Can you work these out from the drawing? Everything is in mm from the part's minimum corner. Round coordinates to 2 decimals unless told otherwise and drop trailing zeros. Write each loop counter-clockwise with the first axis right and the second up, starting at its lowest first coordinate (ties: lowest second). Pieces come first, ordered by that corner, then holes. Notation, with made-up numbers: (28.5, -6) -> (80.5, -6) arc R28 ccw to (80.5, 32) -> close; hole circle Ø11 at (82, 16.25). An arc over 180 degrees is marked (long way). One line per question, with ' | ' between items. Start each with the question number.
1. Imagine slicing it at B-B, the plane y = 5.75. List the corners of the cut face in (x, z) for me.
2. For pin 1 Ø4 at (x, y) = (10.5, 6.5) entering from +Z, with a flat end and sliding along its axis, tell me the tip position at first contact or that it passes through.
3. If I drill on line 1 along X through (y, z) = (6.25, 0.65) (1 decimal); line 2 along Y through (x, z) = (6.25, 0.7) (1 decimal); line 3 along X through (y, z) = (5, 0.6), over which ranges is the centre line in solid material (lowest first)? Write a range as [from, to].
4. Imagine slicing it at C-C, the plane x = 6.5. List the corners of the cut face in (y, z) for me.
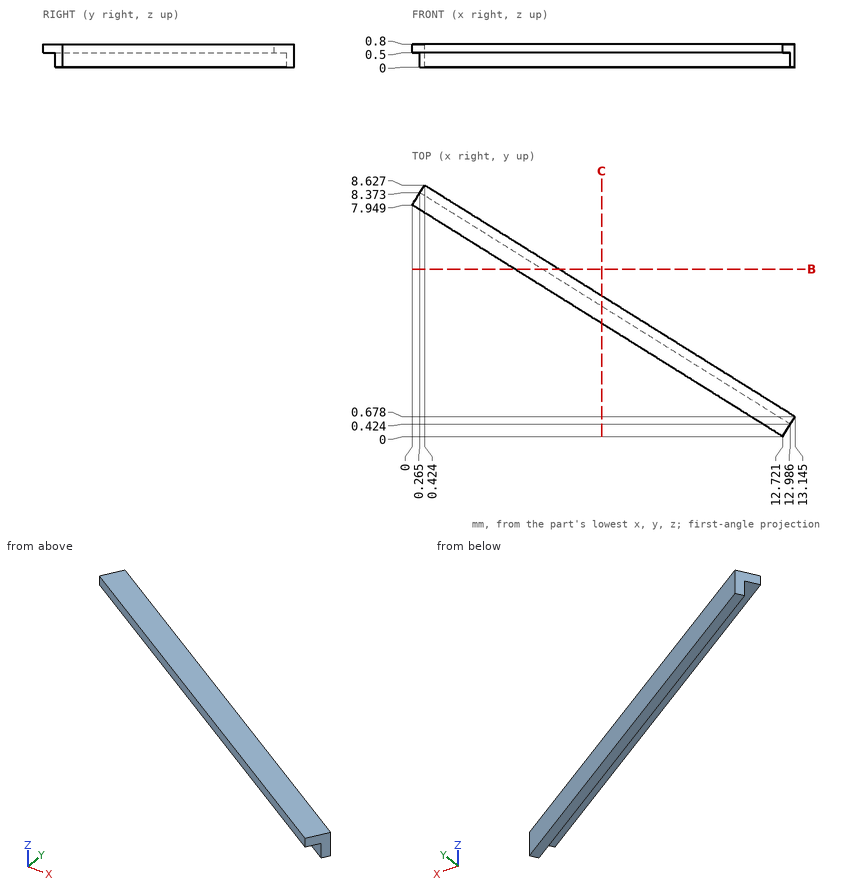
Geometry results:
1) outline: (3.52, 0.5) -> (4.46, 0.5) -> (4.46, 0) -> (5.03, 0) -> (5.03, 0.8) -> (3.52, 0.8) -> close
2) pin 1: passes through
3) line 1: x = [2.7, 4.2] | line 2: y = [4, 5] | line 3: x = [4.72, 6.23]
4) outline: (3.89, 0.5) -> (4.48, 0.5) -> (4.48, 0) -> (4.83, 0) -> (4.83, 0.8) -> (3.89, 0.8) -> close
